For this review, take the finished solid that the model builds, in its own axes (mm). A direction names the side the tool comes from. Give positions to 0.01 mm unless a question says otherwise; leave off trailing zeros. Loops run counter-clockwise (first coordinate to the right, second up) from the corner with the lowest first, then second, coordinate; pieces in that order, holes last.
```python
from build123d import *

# Parameters (mm, degrees)
SKETCH4_R               = 8.5
SKETCH5_R               = 7.5
CUT_EXTRUDE1_DEPTH      = 10
CUT_EXTRUDE1_DEPTH_BACK = 10
SKETCH7_W               = 13.763410073
SKETCH7_H               = 8.5
CUT_EXTRUDE4_DEPTH      = 10
CUT_EXTRUDE4_DEPTH_BACK = 10
CUT_EXTRUDE5_DEPTH      = 10
CUT_EXTRUDE5_DEPTH_BACK = 10
SKETCH11_R              = 1.25
CUT_EXTRUDE6_DEPTH      = 26.069902429
FILLET1_R               = 1


with BuildPart() as part:
    # Sketch4 → Loft1 section 0
    with BuildSketch(Plane(origin=(0, 0, 0), x_dir=(0, 0, -1), z_dir=(1, 0, 0))):
        Circle(SKETCH4_R)
    # Sketch5 → Loft1 section 1
    with BuildSketch(Plane(origin=(22, 0, 0), x_dir=(0, 0, -1), z_dir=(1, 0, 0))):
        Circle(SKETCH5_R)
    loft()

    # Sketch7 → Cut-Extrude1 (cut, two sides: drawn at the far end of the back side and taken through both)
    with BuildSketch(Plane.XY.offset(-CUT_EXTRUDE1_DEPTH_BACK)):
        with Locations((17.881705037, 0)):
            Rectangle(SKETCH7_W, SKETCH7_H)
    extrude(amount=CUT_EXTRUDE1_DEPTH + CUT_EXTRUDE1_DEPTH_BACK, mode=Mode.SUBTRACT)

    # Sketch8 → Cut-Extrude4 (cut, two sides: drawn at the far end of the back side and taken through both)
    with BuildSketch(Plane(origin=(0, 0, 0), x_dir=(1, 0, 0), z_dir=(0, 1, 0)).offset(-CUT_EXTRUDE4_DEPTH_BACK)):
        with BuildLine():
            Line((11, 6.777720856), (16.53, 6.685056145))
            ThreePointArc((16.53, 6.685056145), (21.20100697, 3.731621267), (23, -1.493769414))
            Line((23, -1.493769414), (23, -6.043769414))
            Line((23, -6.043769414), (11, -6.777720856))
            Line((11, -6.777720856), (11, -9.08468988))
            Line((11, -9.08468988), (27.197187836, -9.08468988))
            Line((27.197187836, -9.08468988), (27.197187836, 11.602386845))
            Line((27.197187836, 11.602386845), (11, 11.602386845))
            Line((11, 11.602386845), (11, 6.777720856))
        make_face()
    extrude(amount=CUT_EXTRUDE4_DEPTH + CUT_EXTRUDE4_DEPTH_BACK, mode=Mode.SUBTRACT)

    # Sketch11 → Cut-Extrude5 (cut, two sides: drawn at the far end of the back side and taken through both)
    with BuildSketch(Plane(origin=(0, 0, 0), x_dir=(1, 0, 0), z_dir=(0, 1, 0)).offset(-CUT_EXTRUDE5_DEPTH_BACK)):
        with Locations(Location((15.3, 0.5, 0), (0, 0, 136.441515333))):
            Circle(SKETCH11_R)
    extrude(amount=CUT_EXTRUDE5_DEPTH + CUT_EXTRUDE5_DEPTH_BACK, mode=Mode.SUBTRACT)

    # Sketch12 → Cut-Extrude6 (cut, through all)
    with BuildSketch(Plane.ZY):
        with BuildLine():
            Line((-4.5, 4.25), (4.5, 4.25))
            ThreePointArc((4.5, 4.25), (5.448066505, 0), (4.5, -4.25))
            Line((4.5, -4.25), (-4.5, -4.25))
            ThreePointArc((-4.5, -4.25), (-5.448066505, 0), (-4.5, 4.25))
        make_face()
    extrude(amount=-CUT_EXTRUDE6_DEPTH, mode=Mode.SUBTRACT)

    # Fillet1
    fillet1_edges = [part.edges().sort_by_distance(p)[0] for p in [
        (22, -4.303290893, 6.104932034),
        (22, 4.303290893, 6.104932034),
    ]]
    fillet(fillet1_edges, radius=FILLET1_R)


solid = part.part
```
Q1. Consider section A-A on z = 0. Give the boundary of the cut face in (x, y).
Answers:
outline: (0, -8.5) - (14.15, -7.86) - (14.15, -4.25) - (0, -4.25) - close; (0, 4.25) - (14.15, 4.25) - (14.15, 7.86) - (0, 8.5) - close; (16.45, -7.75) - (22, -7.5) - (22, -4.25) - (16.45, -4.25) - close; (16.45, 4.25) - (22, 4.25) - (22, 7.5) - (16.45, 7.75) - close
Q2. Machinability: for faces 1 (the flat face through (11, 0, 6)), 2 (the flat face through (11, 4.25, 0)), 3 (the cylindrical face through (5.423, 0.061, 5.448)), which of the approach directions +Z, -Z, +X, -X, +Y, -Y give a long, thin tool a straight path to every point of the face, cutting with its end or side? Answer none if there is none.
Answers:
face 1: +Z, -Z, +X
face 2: +X
face 3: +X, -X
Q3. For probe 1 along X at (y, z) = (5.1, -0.5); probe 2 along X at (y, z) = (-1.75, -6.5); probe 3 along Y at (x, z) = (15, -6), list the stretches that pass through material, from the lowest coordinate up.
Answers:
probe 1: x = 0 to 14.05, 16.55 to 22
probe 2: x = 0 to 11
probe 3: y = -5.01 to -4.25, 4.25 to 5.01
Q4. For pin 1 Ø4 at (x, y) = (11.5, -3.5) entering from +Z; pin 2 Ø8 at (x, z) = (7.5, -3) entering from -Y; pin 3 Ø2 at (x, z) = (18.5, -6.5) entering from +Y; pin 4 Ø3 at (y, z) = (-0.5, 3.5) entering from +X, all flat-tipped, find the tip position at first contact; note any pin that passes through.
Answers:
pin 1: stops at z = 7.85
pin 2: stops at y = -8.29
pin 3: stops at y = 5.33
pin 4: passes through
Q5. Consider section C-C on x = 10.5. Give the boundary of the cut face in (y, z).
Answers:
outline: circle Ø16.05 at (0, 0); hole (-4.25, -4.5) arc R10 ccw to (4.25, -4.5) - (4.25, 4.5) arc R10 ccw to (-4.25, 4.5) - close
Q6. Consider section B-B on x = 15. Give the boundary of the cut face in (y, z).
Answers:
outline: (-7.79, 0.71) - (-4.25, 0.71) - (-4.25, 6.53) - (-4.29, 6.53) arc R7.82 ccw to start; (-7.63, -1.71) arc R7.82 ccw to (-4.25, -6.56) - (-4.25, -1.71) - close; (4.25, -6.56) arc R7.82 ccw to (7.63, -1.71) - (4.25, -1.71) - close; (4.25, 0.71) - (7.79, 0.71) arc R7.82 ccw to (4.29, 6.53) - (4.25, 6.53) - close
Q7. Mouldability with a two-part tool opening along Y and no side actions: class faces 4 (the conical face through (11.154, -4.864, 6.343)), 5 (the cylindrical face through (5.423, -0.061, -5.448)), 6 (the flat face through (11, -4.25, 0)), 7 (the flat face through (0, -6, 0)) as +Y half, -Y half, draft (parallel to the pull), parting line (faces both ways), or undercut.
Answers:
face 4: parting line
face 5: undercut
face 6: undercut
face 7: draft
